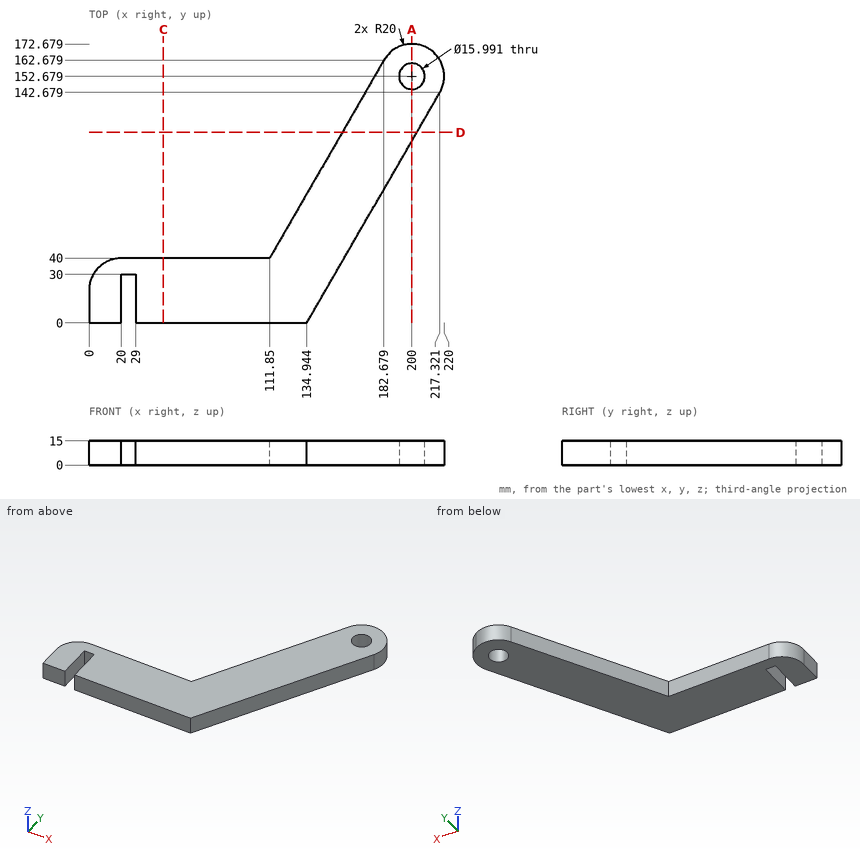
Input: dimensioned drawing with shaded views. Units: mm. Origin: part minimum x, y, z. Coordinates: 2 decimals unless noted, no trailing zeros. Order: outer loops, then holes, each group sorted by start corner. A loop starts at its lowest first (then second) coordinate and runs counter-clockwise, first axis right, second up. Notation, with made-up numbers: (-38, 44) - (14, 44) arc R23 cw to (14, 60) - close; hole circle Ø4 at (29, 60). An arc over 180 degrees is marked (long way). One line per item, written item: value.
1) Cut plane D-D on y = 118. Output: boundary loops of the cut face in (x, z).
Computed values:
outline: (156.88, 0) - (203.07, 0) - (203.07, 15) - (156.88, 15) - close
2) Cut plane A-A on x = 200. Output: boundary loops of the cut face in (y, z) (1 decimal).
Computed values:
outline: (112.7, 0) - (144.7, 0) - (144.7, 15) - (112.7, 15) - close; (160.7, 0) - (172.7, 0) - (172.7, 15) - (160.7, 15) - close
3) Cut plane C-C on x = 46. Output: boundary loops of the cut face in (y, z).
Computed values:
outline: (0, 0) - (40, 0) - (40, 15) - (0, 15) - close
4) Contact query for flat-ended pins moving along their axis: pin 1 (5 mm diameter, centred on x = 85.5, z = 5.5, fed in from +Y); pin 2 (2.5 mm diameter, centred on x = 24.5, z = 7.5, fed in from -Y); pin 3 (4.5 mm diameter, centred on y = 19.5, z = 9.5, fed in from +X); pin 4 (2 mm diameter, centred on x = 47.5, y = 25, fed in from -Z). Output: stop coordinate, or through.
Computed values:
pin 1: stops at y = 40
pin 2: stops at y = 30
pin 3: stops at x = 147.5
pin 4: stops at z = 0
5) Ray query, line 1 (Y direction, x = 24, z = 7); line 2 (X direction, y = 147, z = 5.5) (1 decimal); line 3 (X direction, y = 152, z = 10.5) (1 decimal). Return the intervals inside material, ascending. Write a range as [from, to].
Computed values:
line 1: y = [30, 40]
line 2: x = [173.6, 194.4], [205.6, 219.2]
line 3: x = [176.5, 192], [208, 220]
